Source: CAD feature listing. Evaluate the final solid. Frame: model axes, mm. A direction names the side the tool comes from. Coordinates: 2 decimals unless noted, no trailing zeros. Loops run counter-clockwise (first coordinate to the right, second up) from the corner with the lowest first, then second, coordinate; pieces in that order, holes last. Notation, with made-up numbers: (-19.75, -28.75) - (28.25, -28.75) arc R14 cw to (28.25, -2.75) - close; hole circle Ø11 at (-38.75, 84). An arc over 180 degrees is marked (long way). Use one line per item in the form item = value. Start each with the question number.
Autodesk Inventor part; units mm, degrees
ref_plane "YZ Plane" through (0, 0, 0) normal (1, 0, 0) x (0, 1, 0)
ref_plane "XZ Plane" through (0, 0, 0) normal (0, 1, 0) x (-1, 0, 0)
ref_plane "XY Plane" through (0, 0, 0) normal (0, 0, 1) x (1, 0, 0)
sketch "Sketch1" plane through (0, 0, 0) normal (0, 1, 0) x (-1, 0, 0)
  arc A0 (1.5943, -9.3653) -> (-1.5943, -9.3653) centre (0, -9.5) ccw
  arc A1 (8.9077, -3.3019) -> (7.3134, -6.0634) centre (8.2272, -4.75) ccw
  arc A2 (7.3134, 6.0634) -> (8.9077, 3.3019) centre (8.2272, 4.75) ccw
  arc A3 (-1.5943, 9.3653) -> (1.5943, 9.3653) centre (0, 9.5) ccw
  arc A4 (-8.9077, 3.3019) -> (-7.3134, 6.0634) centre (-8.2272, 4.75) ccw
  arc A5 (-7.3134, -6.0634) -> (-8.9077, -3.3019) centre (-8.2272, -4.75) ccw
  arc A6 (1.5943, -9.3653) -> (7.3134, -6.0634) centre (0, 0) ccw
  arc A7 (8.9077, -3.3019) -> (8.9077, 3.3019) centre (0, 0) ccw
  arc A8 (7.3134, 6.0634) -> (1.5943, 9.3653) centre (0, 0) ccw
  arc A9 (-1.5943, 9.3653) -> (-7.3134, 6.0634) centre (0, 0) ccw
  arc A10 (-8.9077, 3.3019) -> (-8.9077, -3.3019) centre (0, 0) ccw
  arc A11 (-7.3134, -6.0634) -> (-1.5943, -9.3653) centre (0, 0) ccw
  dimension "d1" = 3.2
  dimension "d4" = 360
extrude "Extrusion1" add sketch "Sketch1" along normal blind 2
sketch "Sketch2" plane through (0, 2, 0) normal (0, 1, 0) x (1, 0, 0)
  line L0 (2, 2) -> (-2, 2)
  line L1 (-2, 2) -> (-2, -2)
  line L2 (-2, -2) -> (2, -2)
  line L3 (2, -2) -> (2, 2)
  line L4 (2, 2) -> (-2, -2) construction
  line L5 (-2, 2) -> (2, -2) construction
  point P0 (0, 0)
  dimension "d8" = 4
  dimension "d9" = 4
extrude "Extrusion2" add sketch "Sketch2" along normal blind 2
properties part number "led"
(1) Access query for faces 4 (the face through (0, 3, -2)), 5 (the face through (-9.5, 1, 0)), 6 (the face through (-2, 3, 0)), 7 (the face through (2, 3, 0)), 8 (the face through (0, 3, 2)). Directions: +Z, -Z, +X, -X, +Y, -Y. A direction counts if a zero-diameter tool reaches every point of the face in a straight line with its end or side. Return the directions, or none.
(2) Mould query, pull axis Z, two halves, no side actions, for faces 1 (the face through (4.8, 1, 8.2)), 2 (the face through (0, 1, -7.9)), 3 (the face through (-6.86, 0.99, 3.92)). Classes: +Z half, -Z half, draft (parallel to the pull), parting line (faces both ways), or undercut.
(3) Cut plane C-C, the plane z = -1.75. Output: boundary loops of the cut face in (x, y), plus the area to 3 significant figures.
(4) Cut plane A-A, the plane y = 1.65. Output: boundary loops of the cut face in (x, z), plus the area to 3 significant figures.
(5) Contact query for flat-ended pins moving along their axis: pin 1 (1.6 mm diameter, centred on x = 0.5, y = 3, fed in from -Z); pin 2 (3 mm diameter, centred on x = 0.5, z = -5, fed in from +Y); pin 3 (1.6 mm diameter, centred on y = 3.5, z = 0.5, fed in from -X); pin 4 (1.5 mm diameter, centred on y = 3, z = -3.5, fed in from +X). Output: stop coordinate, or through.
(6) Cut plane B-B, the plane x = -0.5. Output: boundary loops of the cut face in (y, z), plus the area to 3 significant figures.
(7) Cut plane D-D, the plane y = 3.6. Output: boundary loops of the cut face in (x, z).
(8) Material intervals for line 1 (Z direction, x = 7, y = 1.8); line 2 (Z direction, x = 1.75, y = 2.05); line 3 (Y direction, x = -4.75, z = 3.75), sorted ascending.
Recorded:
q1.face_4 = -Z, +X, -X, +Y
q1.face_5 = -X, +Y, -Y
q1.face_6 = +Z, -Z, -X, +Y
q1.face_7 = +Z, -Z, +X, +Y
q1.face_8 = +Z, +X, -X, +Y
q2.face_1 = +Z half
q2.face_2 = -Z half
q2.face_3 = undercut
q3.outline = (-9.34, 0) - (9.34, 0) - (9.34, 2) - (2, 2) - (2, 4) - (-2, 4) - (-2, 2) - (-9.34, 2) - close
q3.area = 45.3 mm²
q4.outline = (-8.91, -3.3) arc R1.6 cw to (-7.31, -6.06) arc R9.5 ccw to (-1.59, -9.37) arc R1.6 cw to (1.59, -9.37) arc R9.5 ccw to (7.31, -6.06) arc R1.6 cw to (8.91, -3.3) arc R9.5 ccw to (8.91, 3.3) arc R1.6 cw to (7.31, 6.06) arc R9.5 ccw to (1.59, 9.37) arc R1.6 cw to (-1.59, 9.37) arc R9.5 ccw to (-7.31, 6.06) arc R1.6 cw to (-8.91, 3.3) arc R9.5 ccw to start
q4.area = 260 mm²
q5.pin_1 = -2
q5.pin_2 = 2
q5.pin_3 = -2
q5.pin_4 = through
q6.outline = (0, -7.98) - (2, -7.98) - (2, -2) - (4, -2) - (4, 2) - (2, 2) - (2, 7.98) - (0, 7.98) - close
q6.area = 39.9 mm²
q7.outline = (-2, -2) - (2, -2) - (2, 2) - (-2, 2) - close
q8.line_1 = -6.42 to -5.78, -3.72 to 3.72, 5.78 to 6.42
q8.line_2 = -2 to 2
q8.line_3 = 0 to 2
